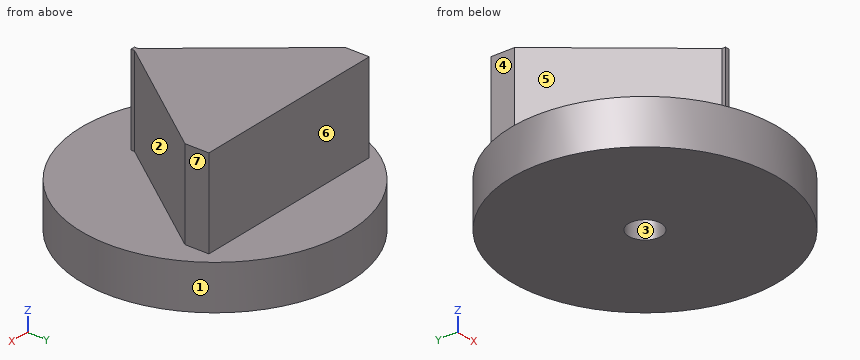
from build123d import *

# Parameters (mm, degrees)
F1_DEPTH   = 25.4
F2_W       = 112.7116382122
F2_H       = 13.5166756809
F2_W_2     = 2.3981197737
F2_H_2     = 1.962095499
F3_DEPTH   = 25.4
F3_FACE_W  = 112.7116382122
F3_FACE_H  = 25.4
F3_FACE1_W = 2.3981197737
F3_FACE1_H = 25.4
F5_DEPTH   = 25.4


with BuildPart() as f1:
    # F0 (on Top) → F1 (new body)
    with BuildSketch(Plane.XY):
        with BuildLine():
            Line((9.2957576653, 0), (75.818580382, 0))
            ThreePointArc((75.818580382, 0), (0, 75.818580382), (-75.818580382, 0))
            Line((-75.818580382, 0), (-9.2957576653, 0))
            ThreePointArc((-9.2957576653, 0), (0, 9.2957576653), (9.2957576653, 0))
        make_face()
        with BuildLine():
            ThreePointArc((-75.818580382, 0), (0, -75.818580382), (75.818580382, 0))
            Line((75.818580382, 0), (9.2957576653, 0))
            ThreePointArc((9.2957576653, 0), (0, -9.2957576653), (-9.2957576653, 0))
            Line((-9.2957576653, 0), (-75.818580382, 0))
        make_face()
    extrude(amount=F1_DEPTH)

    # F2 (on face) → F3 (join)
    with BuildSketch(Plane.XY.offset(25.4)):
        with Locations((-1.6350820661, 33.7916892022)):
            Rectangle(F2_W, F2_H)
        with Locations((1.1990598869, -44.5832274854)):
            Rectangle(F2_W_2, F2_H_2)
    extrude(amount=F3_DEPTH)

    # F3_face (on face) → F4 section 0
    with BuildSketch(Plane(origin=(-1.6350820661, 27.0333513618, 38.1), x_dir=(1, 0, 0), z_dir=(0, -1, 0))):
        Rectangle(F3_FACE_W, F3_FACE_H)
    # F3_face1 (on face) → F4 section 1
    with BuildSketch(Plane(origin=(1.1990598869, -43.6021797359, 38.1), x_dir=(-1, 0, 0), z_dir=(0, 1, 0))):
        Rectangle(F3_FACE1_W, F3_FACE1_H)
    loft()

    # F5 (add): a face of the model
    f5_faces = [f1.faces().sort_by_distance(p)[0] for p in [
        (-0.9317783137, 11.344748031, 50.8),
    ]]
    extrude(f5_faces, amount=F5_DEPTH)


solid = f1.part
The listing builds one solid part. Answer for the finished solid, in the listing's coordinates (mm). Face numbers are marked on the shaded views. A direction names the side the tool comes from. Give positions to 0.01 mm unless a question says otherwise; leave off trailing zeros. Order: outer loops, then holes, each group sorted by start corner. A loop starts at its lowest first (then second) coordinate and runs counter-clockwise, first axis right, second up. Notation, with made-up numbers: (0, 36.5) -> (15, 36.5) arc R18 ccw to (15, 43.5) -> close; hole circle Ø3 at (48.25, 8). An arc over 180 degrees is marked (long way). Put each result on its own line as item: value.
Item 1: For the marked faces 5, 6 and 7, determine the directions among +Z, -Z, +X, -X, +Y, -Y from which every point of the face is accessible in a straight line to the end or side of a thin tool.
Established:
face 5: +Z, -X, -Y
face 6: +Z, +X, -X, +Y
face 7: +Z, +X, +Y, -Y
Item 2: A cutting plane is placed at D-D on y = -49.5. Give the vertices of the cut face in (x, z).
Established:
outline: (-57.43, 0) -> (57.43, 0) -> (57.43, 25.4) -> (-57.43, 25.4) -> close
Item 3: A cutting plane is placed at A-A on z = 65. Give the vertices of the cut face in (x, y).
Established:
outline: (-57.99, 27.03) -> (0, -43.6) -> (0, -45.56) -> (2.4, -45.56) -> (2.4, -43.6) -> (54.72, 27.03) -> (54.72, 40.55) -> (-57.99, 40.55) -> close
Item 4: For a pull along X with two mould halves and no side action, classify the marked faces 1, 2, 3 and 4 as released by +X, released by -X, zero draft, split by the parting line, or undercut.
Established:
face 1: split by the parting line
face 2: released by +X
face 3: undercut
face 4: released by -X
Item 5: A cutting plane is placed at C-C on z = 8.5. Give the vertices of the cut face in (x, y), plus the area to 3 significant figures.
Established:
outline: circle Ø151.64 at (0, 0); hole circle Ø18.59 at (0, 0)
area: 17,800 mm^2
Item 6: Straight lines are drawn through the part: line 1 (Y direction, x = 0, z = 10); line 2 (Z direction, x = -56, y = 48); line 3 (X direction, y = -7, z = 8.5). For each, find the intervals that lie inside material, in ascending order.
Established:
line 1: y = -75.82 to -9.3, 9.3 to 75.82
line 2: z = 0 to 25.4
line 3: x = -75.49 to -6.12, 6.12 to 75.49
Item 7: Given P1, Ø4, axis at y = -57, z = 12, coming from the -X side; P2, Ø11, axis at y = 31.5, z = 51.5, coming from the -X side; P3, Ø15, axis at x = -9.5, z = 60, coming from the +Y side, each flat-ended and moving along its own axis, determine where each tip first touches the part or whether it passes through.
Established:
P1: stops at x = -52.19
P2: stops at x = -57.99
P3: stops at y = 40.55
Item 8: A cutting plane is placed at B-B on x = 31. Give the vertices of the cut face in (y, z), plus the area to 3 significant figures.
Established:
outline: (-69.19, 0) -> (69.19, 0) -> (69.19, 25.4) -> (40.55, 25.4) -> (40.55, 76.2) -> (-4.99, 76.2) -> (-4.99, 25.4) -> (-69.19, 25.4) -> close
area: 5,830 mm^2
